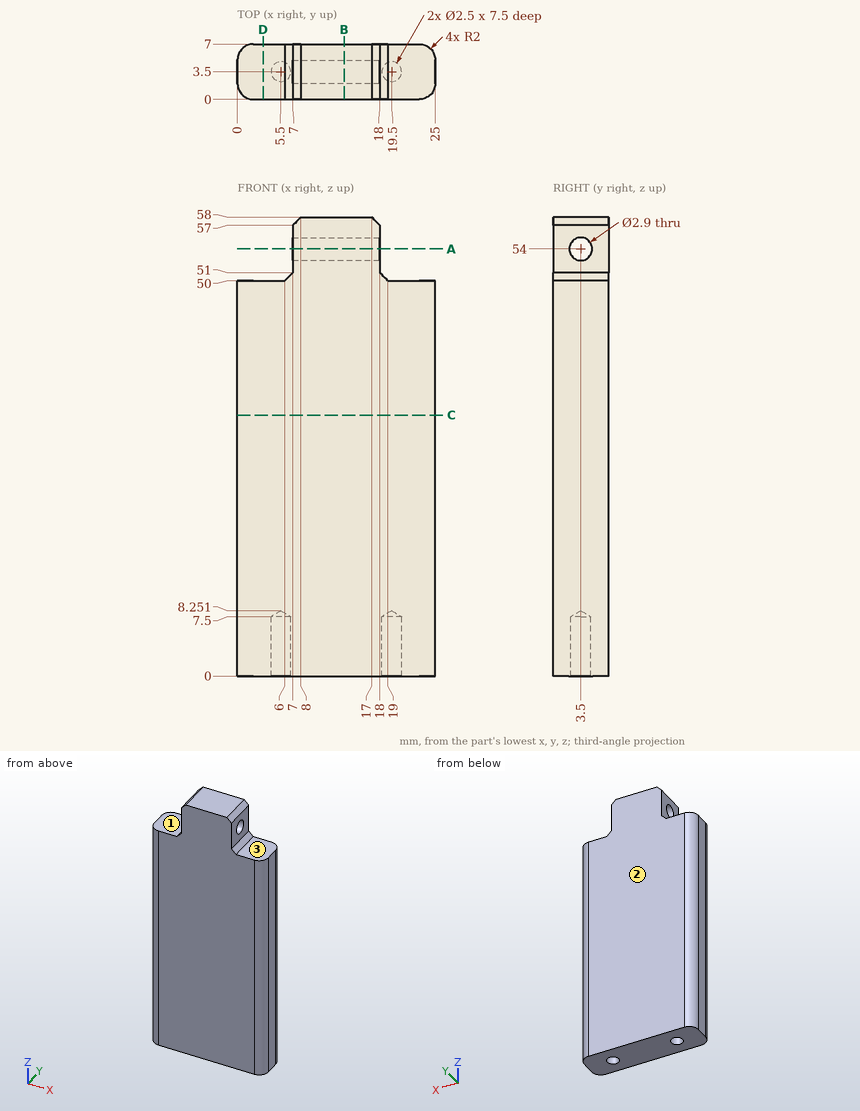
Geometry check sheet. Reference: drawing and pictorial views, mm from the part's lowest x, y, z. A direction names the side the tool comes from. Round coordinates to 2 decimals unless told otherwise and drop trailing zeros. Loops run counter-clockwise (first coordinate to the right, second up) from the corner with the lowest first, then second, coordinate; pieces in that order, holes last. Notation, with made-up numbers: (69, -17) - (78, -17) arc R17 cw to (78, -5) - close; hole circle Ø8 at (-7.75, -31). An arc over 180 degrees is marked (long way). Answer in a Markdown table with one row per item. Add a question column.
Q1. Section check D-D on x = 3.25. Enter the section's corners in (y, z).
Q2. Tool access check on the marked faces 1, 2 and 3. Record the directions out of +Z, -Z, +X, -X, +Y, -Y that give a thin tool (end or side, any length) a straight path to the whole face; none if there is none.
Q3. Material ranges on line 1 (X direction, y = 3.5, z = 5); line 2 (Y direction, x = 19.5, z = 5.25); line 3 (Z direction, x = 3.25, y = 6.5), recorded low to high.
Q4. Section check A-A on z = 54. Enter the section's corners in (x, y), plus the area to 3 significant figures.
Q5. Gauge pin test, flat ends, axial feed: pin 1 (1.5 mm diameter, centred on x = 19.5, y = 3.5, fed in from -Z); pin 2 (3.5 mm diameter, centred on y = 3.5, z = 54, fed in from +X); pin 3 (3 mm diameter, centred on x = 22.5, y = 3, fed in from +Z). Record the tip position at first contact, or that the pin passes through.
Q6. Section check B-B on x = 13.5. Enter the section's corners in (y, z).
Q7. Section check C-C on z = 33. Enter the section's corners in (x, y), plus the area to 3 significant figures.
Found:
| question | item | result |
|---|---|---|
| 1 | outline | (0, 0) - (7, 0) - (7, 50) - (0, 50) - close |
| 2 | face 1 | +Z, -X, +Y, -Y |
| 2 | face 2 | +Z, -Z, +X, -X, +Y |
| 2 | face 3 | +Z, +X, +Y, -Y |
| 3 | line 1 | x = 0 to 4.25, 6.75 to 18.25, 20.75 to 25 |
| 3 | line 2 | y = 0 to 2.25, 4.75 to 7 |
| 3 | line 3 | z = 0 to 50 |
| 4 | outline | (7, 0) - (18, 0) - (18, 2.05) - (7, 2.05) - close; (7, 4.95) - (18, 4.95) - (18, 7) - (7, 7) - close |
| 4 | area | 45.1 mm² |
| 5 | pin 1 | stops at z = 7.8 |
| 5 | pin 2 | stops at x = 18 |
| 5 | pin 3 | stops at z = 50 |
| 6 | outline | (0, 0) - (7, 0) - (7, 58) - (0, 58) - close; hole circle Ø2.9 at (3.5, 54) |
| 7 | outline | (0, 2) arc R2 ccw to (2, 0) - (23, 0) arc R2 ccw to (25, 2) - (25, 5) arc R2 ccw to (23, 7) - (2, 7) arc R2 ccw to (0, 5) - close |
| 7 | area | 172 mm² |
